```python
from build123d import *

# Parameters (mm, degrees)
SKETCH_R        = 8.5
PAD_DEPTH       = 1.5
SKETCH001_R     = 4
SKETCH001_R_2   = 1.15
POCKET_DEPTH    = 5
SKETCH002_W     = 6
SKETCH002_H     = 14
PAD001_DEPTH    = 6
SKETCH003_R     = 1.15
POCKET001_DEPTH = 15


with BuildPart() as part:
    # Sketch → Pad (new body)
    with BuildSketch(Plane.XY):
        Circle(SKETCH_R)
    extrude(amount=PAD_DEPTH)

    # Sketch001 → Pocket (cut)
    with BuildSketch(Plane.XY.offset(1.5)):
        Circle(SKETCH001_R)
        with Locations((-6, 0)):
            Circle(SKETCH001_R_2)
        with Locations((6, 0)):
            Circle(SKETCH001_R_2)
    extrude(amount=-POCKET_DEPTH, mode=Mode.SUBTRACT)

    # Sketch002 → Pad001 (new body)
    with BuildSketch(Plane(origin=(0, 0, 0), x_dir=(1, 0, 0), z_dir=(0, 0, -1))):
        with Locations((0, 11)):
            Rectangle(SKETCH002_W, SKETCH002_H)
    extrude(amount=-PAD001_DEPTH)

    # Sketch003 → Pocket001 (cut)
    with BuildSketch(Plane.XZ.offset(18)):
        with Locations((0, 3)):
            Circle(SKETCH003_R)
    extrude(amount=-POCKET001_DEPTH, mode=Mode.SUBTRACT)


solid = part.part
```
Check sheet for the modelled part. Datum: model origin and axes. Units: mm. A direction names the side the tool comes from. Round coordinates to 2 decimals unless told otherwise and drop trailing zeros. Write each loop counter-clockwise with the first axis right and the second up, starting at its lowest first coordinate (ties: lowest second). Pieces come first, ordered by that corner, then holes. Notation, with made-up numbers: M 46,24 L 90,24 A30 ccw 90,57 Z; hole C 47,86.5 d5. An arc over 180 degrees is marked long. Write item = value, one per line. Start each with the question number.
1. Section check B-B, the plane z = 3.4. Record the cut outline in (x, y), then the cut area to 3 significant figures.
2. Gauge pin test, flat ends, axial feed: pin 1 (1 mm diameter, centred on y = -13.5, z = 2, fed in from +X); pin 2 (3 mm diameter, centred on x = 6, y = 0, fed in from +Z); pin 3 (1.5 mm diameter, centred on x = 6, z = 4, fed in from +Y); pin 4 (2 mm diameter, centred on x = 0.5, z = 4, fed in from +Y). Record the tip position at first contact, or that the pin passes through.
3. Section check A-A, the plane y = 0. Record the cut outline in (x, z).
4. Section check D-D, the plane y = -12.25. Record the cut outline in (x, z), then the cut area to 3 significant figures.
5. Scan lines: line 1 (Y direction, x = -1.5, z = 1.6); line 2 (X direction, y = -16.5, z = 0.9); line 3 (Y direction, x = -6, z = 1.1). Record each from-to range of solid material in increasing order. Write a range as [from, to].
6. Tool access check on faces 5 (the cylindrical face through (0.331, 8.494, 0.74)), 6 (the flat face through (3, -11, 3)), 7 (the flat face through (-3, -11, 3)). Record the directions out of +Z, -Z, +X, -X, +Y, -Y that give a thin tool (end or side, any length) a straight path to the whole face; none if there is none.
7. Release check for a two-part mould opening along Y. For faces 1 (the cylindrical face through (-0.867, -3.905, 0.76)), 2 (the flat face through (1, -4, 4)), 3 (the cylindrical face through (4.85, 0.05, 0.76)), 4 (the flat face through (2, 4, 1.5)) record: pulls with the +Y half, pulls with the -Y half, needs draft (parallel to the pull), parting line crosses it, or undercut.
8. Section check C-C, the plane x = 6. Record the cut outline in (y, z), then the cut area to 3 significant figures.
Results found:
q1.outline = M -3,-18 L -1.08,-18 L -1.08,-4 L -3,-4 Z; M 1.08,-18 L 3,-18 L 3,-4 L 1.08,-4 Z
q1.area = 53.8 mm^2
q2.pin_1 = 3
q2.pin_2 = 1.5
q2.pin_3 = through
q2.pin_4 = -4
q3.outline = M -8.5,0 L -7.15,0 L -7.15,1.5 L -8.5,1.5 Z; M -4.85,0 L -4,0 L -4,1.5 L -4.85,1.5 Z; M 4,0 L 4.85,0 L 4.85,1.5 L 4,1.5 Z; M 7.15,0 L 8.5,0 L 8.5,1.5 L 7.15,1.5 Z
q4.outline = M -3,0 L 3,0 L 3,6 L -3,6 Z; hole C 0,3 d2.3
q4.area = 31.8 mm^2
q5.line_1 = [-18, -4]
q5.line_2 = [-3, 3]
q5.line_3 = [-6.02, -1.15], [1.15, 6.02]
q6.face_5 = +Z, -Z
q6.face_6 = +Z, +X, -Y
q6.face_7 = +Z, -X, -Y
q7.face_1 = undercut
q7.face_2 = pulls with the +Y half
q7.face_3 = undercut
q7.face_4 = needs draft
q8.outline = M -6.02,0 L -1.15,0 L -1.15,1.5 L -6.02,1.5 Z; M 1.15,0 L 6.02,0 L 6.02,1.5 L 1.15,1.5 Z
q8.area = 14.6 mm^2
